```python
from build123d import *

# Parameters (mm, degrees)
SKETCH_1_W      = 49
SKETCH_1_H      = 32
SKETCH_1_R      = 6
EXTRUDE_1_DEPTH = 20
SKETCH_3_W      = 49
SKETCH_3_H      = 59
EXTRUDE_2_DEPTH = 20
FILLET_1_R      = 10
FILLET_2_R      = 5
FILLET_3_R      = 5
FILLET_4_R      = 5


with BuildPart() as part:
    # 草图1 → 凸台-拉伸1 (new body)
    with BuildSketch(Plane(origin=(0, 0, 0), x_dir=(1, 0, 0), z_dir=(0, 1, 0))):
        Rectangle(SKETCH_1_W, SKETCH_1_H)
        with Locations(Location((0, 0, 0), (0, 0, 270))):
            Circle(SKETCH_1_R, mode=Mode.SUBTRACT)
    extrude(amount=EXTRUDE_1_DEPTH)

    # 草图3 → 凸台-拉伸2 (add)
    # profile 1 of 2: a face of its own
    with BuildSketch(Plane(origin=(0, 0, 0), x_dir=(1, 0, 0), z_dir=(0, 1, 0))):
        with Locations((0, 45.5)):
            Rectangle(SKETCH_3_W, SKETCH_3_H)
        with BuildLine():
            ThreePointArc((-7.5, 24), (0, 16.5), (7.5, 24))
            Line((7.5, 24), (7.5, 67))
            ThreePointArc((7.5, 67), (0, 74.5), (-7.5, 67))
            Line((-7.5, 67), (-7.5, 24))
        make_face(mode=Mode.SUBTRACT)
    # profile 2 of 2: a face of its own
    with BuildSketch(Plane(origin=(0, 0, 0), x_dir=(1, 0, 0), z_dir=(0, 1, 0))):
        Polygon((10.5, 108), (24.5, 75), (-24.5, 75), (-10.5, 108), align=None)
    extrude(amount=EXTRUDE_2_DEPTH)

    # 圆角1
    fillet_1_edges = [part.edges().sort_by_distance(p)[0] for p in [
        (-24.5, 10, -75),
        (24.5, 10, -75),
    ]]
    fillet(fillet_1_edges, radius=FILLET_1_R)

    # 圆角2
    fillet_2_edges = [part.edges().sort_by_distance(p)[0] for p in [
        (24.5, 20, -28.483251194),
        (17.102908909, 20, -92.436000428),
        (0, 20, -108),
        (-17.102908909, 0, -92.436000428),
        (-17.102908909, 20, -92.436000428),
        (0, 0, -108),
        (17.102908909, 0, -92.436000428),
        (-24.5, 0, -28.483251194),
        (-24.299443305, 0, -74.959216844),
        (24.299443305, 0, -74.959216844),
        (-24.5, 20, -28.483251194),
        (-24.299443305, 20, -74.959216844),
        (24.299443305, 20, -74.959216844),
        (24.5, 0, -28.483251194),
        (24.5, 10, 16),
        (-24.5, 10, 16),
    ]]
    fillet(fillet_2_edges, radius=FILLET_2_R)

    # 圆角3
    # the kernel refuses this fillet: 5 mm, written as the material it takes off along each edge
    with BuildSketch(Plane(origin=(-19.5, 15, 11), x_dir=(0, 0, 1), z_dir=(0, 1, 0))) as fillet_3_piece_1_section:
        Polygon((0, 0), (FILLET_3_R, 0), (FILLET_3_R, -FILLET_3_R), (0, -FILLET_3_R), align=None)
    fillet_3_piece_1 = extrude(amount=FILLET_3_R, mode=Mode.PRIVATE)
    fillet_3_piece_1 = fillet_3_piece_1 - Plane(origin=(-19.5, 15, 11), x_dir=(0.7071067811865475, 0, -0.7071067811865475), z_dir=(0, 1, 0)) * Sphere(FILLET_3_R, mode=Mode.PRIVATE)
    add(fillet_3_piece_1, mode=Mode.SUBTRACT)
    with BuildSketch(Plane(origin=(19.5, 15, 11), x_dir=(0, 0, 1), z_dir=(0, 1, 0))) as fillet_3_piece_2_section:
        Polygon((0, 0), (FILLET_3_R, 0), (FILLET_3_R, FILLET_3_R), (0, FILLET_3_R), align=None)
    fillet_3_piece_2 = extrude(amount=FILLET_3_R, mode=Mode.PRIVATE)
    fillet_3_piece_2 = fillet_3_piece_2 - Plane(origin=(19.5, 15, 11), x_dir=(-0.7071067811865475, 0, -0.7071067811865475), z_dir=(0, 1, 0)) * Sphere(FILLET_3_R, mode=Mode.PRIVATE)
    add(fillet_3_piece_2, mode=Mode.SUBTRACT)
    with BuildSketch(Plane(origin=(-19.5, 20, 16), x_dir=(0, 0, -1), z_dir=(1, 0, 0))) as fillet_3_piece_3:
        with BuildLine():
            CenterArc((FILLET_3_R, -FILLET_3_R), FILLET_3_R, 90, 90)
            Line((0, -FILLET_3_R), (0, 0))
            Line((0, 0), (FILLET_3_R, 0))
        make_face()
    extrude(amount=39, mode=Mode.SUBTRACT)

    # 圆角4
    # the kernel refuses this fillet: 5 mm, written as the material it takes off along each edge
    with BuildSketch(Plane(origin=(-19.5, 5, 11), x_dir=(0, -1, 0), z_dir=(0, 0, 1))) as fillet_4_piece_1_section:
        Polygon((0, 0), (FILLET_4_R, 0), (FILLET_4_R, -FILLET_4_R), (0, -FILLET_4_R), align=None)
    fillet_4_piece_1 = extrude(amount=FILLET_4_R, mode=Mode.PRIVATE)
    fillet_4_piece_1 = fillet_4_piece_1 - Plane(origin=(-19.5, 5, 11), x_dir=(0.7071067811865475, 0.7071067811865475, 0), z_dir=(0, 0, 1)) * Sphere(FILLET_4_R, mode=Mode.PRIVATE)
    add(fillet_4_piece_1, mode=Mode.SUBTRACT)
    with BuildSketch(Plane(origin=(19.5, 5, 11), x_dir=(0, -1, 0), z_dir=(0, 0, 1))) as fillet_4_piece_2_section:
        Polygon((0, 0), (FILLET_4_R, 0), (FILLET_4_R, FILLET_4_R), (0, FILLET_4_R), align=None)
    fillet_4_piece_2 = extrude(amount=FILLET_4_R, mode=Mode.PRIVATE)
    fillet_4_piece_2 = fillet_4_piece_2 - Plane(origin=(19.5, 5, 11), x_dir=(-0.7071067811865475, 0.7071067811865475, 0), z_dir=(0, 0, 1)) * Sphere(FILLET_4_R, mode=Mode.PRIVATE)
    add(fillet_4_piece_2, mode=Mode.SUBTRACT)
    with BuildSketch(Plane(origin=(-19.5, 0, 16), x_dir=(0, 1, 0), z_dir=(1, 0, 0))) as fillet_4_piece_3:
        with BuildLine():
            CenterArc((FILLET_4_R, -FILLET_4_R), FILLET_4_R, 90, 90)
            Line((0, -FILLET_4_R), (0, 0))
            Line((0, 0), (FILLET_4_R, 0))
        make_face()
    extrude(amount=39, mode=Mode.SUBTRACT)


solid = part.part
```
Design review of the part built by this model. Coordinates are the model's own, in mm. A direction names the side the tool comes from. Give positions to 0.01 mm unless a question says otherwise; leave off trailing zeros. Order: outer loops, then holes, each group sorted by start corner. A loop starts at its lowest first (then second) coordinate and runs counter-clockwise, first axis right, second up. Notation, with made-up numbers: (-36.75, -40) -> (9.25, -40) arc R16 ccw to (9.25, -36) -> close; hole circle Ø4 at (23.25, 3.5). An arc over 180 degrees is marked (long way). Write item = value, one per line. Start each with the question number.
(1) We need section D-D on z = 0. Write out the cut boundary in (x, y).
(2) For faces 1 (the face through (0.16, 9.86, -74.5)), 2 (the face through (0, 19, 14)), list the 3-axis set-ups (+Z, -Z, +X, -X, +Y, -Y) from which the entire face can be reached by the end or side of a thin tool; tool diameter is ignored.
(3) For pin 1 (3 mm diameter, centred on y = 17, z = -13.5, fed in from +X); pin 2 (1 mm diameter, centred on x = 0.5, y = 3, fed in from -Z), all flat-tipped, find the tip position at first contact; note any pin that passes through.
(4) We need section C-C on y = 8. Write out the cut boundary in (x, z), plus the area to 3 significant figures.
(5) We need section A-A on x = 0. Write out the cut boundary in (y, z).
(6) We need section B-B on z = -64. Write out the cut boundary in (x, y), plus the area to 3 significant figures.
(7) Mouldability with a two-part tool opening along X and no side actions: class faces 3 (the face through (-7.5, 10, -46)), 4 (the face through (23, 10.07, 14.57)), 5 (the face through (-0.16, 9.86, -16.5)), 6 (the face through (-15.63, 1.43, -92.07)) as +X half, -X half, draft (parallel to the pull), parting line (faces both ways), or undercut.
(8) To check wall thickness, follow line 1 along X through (y, z) = (4.75, 0); line 2 along Z through (x, y) = (2.5, 2.25); line 3 along Z through (x, y) = (-0.5, 11.75). State the ranges of each line that lie inside material, in increasing order.
Numbers:
q1.outline = (-24.5, 5) arc R5 ccw to (-19.5, 0) -> (-6, 0) -> (-6, 20) -> (-19.5, 20) arc R5 ccw to (-24.5, 15) -> close; (6, 0) -> (19.5, 0) arc R5 ccw to (24.5, 5) -> (24.5, 15) arc R5 ccw to (19.5, 20) -> (6, 20) -> close
q2.face_1 = +Y, -Y
q2.face_2 = +Z, +X, -X, +Y
q3.pin_1 = 24.47
q3.pin_2 = -107.77
q4.outline = (-24.5, -72.97) arc R10 ccw to (-23.71, -76.87) -> (-10.5, -108) -> (10.5, -108) -> (23.71, -76.87) arc R10 ccw to (24.5, -72.97) -> (24.5, 11) arc R5 ccw to (19.5, 16) -> (-19.5, 16) arc R5 ccw to (-24.5, 11) -> close; hole (-7.5, -67) arc R7.5 ccw to (7.5, -67) -> (7.5, -24) arc R7.5 ccw to (-7.5, -24) -> close; hole circle Ø12 at (0, 0)
q4.area = 4,670 mm^2
q5.outline = (0, -103) arc R5 ccw to (5, -108) -> (15, -108) arc R5 ccw to (20, -103) -> (20, -74.5) -> (0, -74.5) -> close; (0, -16.5) -> (20, -16.5) -> (20, -6) -> (0, -6) -> close; (0, 6) -> (20, 6) -> (20, 11) arc R5 ccw to (15, 16) -> (5, 16) arc R5 ccw to (0, 11) -> close
q6.outline = (-24.5, 5) arc R5 ccw to (-19.5, 0) -> (-7.5, 0) -> (-7.5, 20) -> (-19.5, 20) arc R5 ccw to (-24.5, 15) -> close; (7.5, 0) -> (19.5, 0) arc R5 ccw to (24.5, 5) -> (24.5, 15) arc R5 ccw to (19.5, 20) -> (7.5, 20) -> close
q6.area = 659 mm^2
q7.face_3 = undercut
q7.face_4 = +X half
q7.face_5 = undercut
q7.face_6 = -X half
q8.line_1 = -24.49 to -6, 6 to 24.49
q8.line_2 = -107.18 to -74.07, -16.93 to -5.45, 5.45 to 15.18
q8.line_3 = -108 to -74.48, -16.52 to -5.98, 5.98 to 16
